```python
from build123d import *

# Parameters (mm, degrees)
BOSS_EXTRUDE1_DEPTH = 177.8
SKETCH4_W           = 153.979316793
SKETCH4_H           = 25.4
BOSS_EXTRUDE4_DEPTH = 177.8
SKETCH3_R           = 73.2155
CUT_EXTRUDE2_DEPTH  = 25.4
FILLET1_R           = 2.54


with BuildPart() as part:
    # Sketch2 → Boss-Extrude1 (new body)
    with BuildSketch(Plane(origin=(0, 0, 0), x_dir=(1, 0, 0), z_dir=(0, 1, 0))):
        Polygon((0, 0), (153.979316793, 0), (153.979316793, 88.9), align=None)
    extrude(amount=BOSS_EXTRUDE1_DEPTH)

    # Sketch4 → Boss-Extrude4 (add)
    with BuildSketch(Plane(origin=(0, 0, 0), x_dir=(-1, 0, 0), z_dir=(0, -1, 0))):
        with Locations((-76.989658397, -12.7)):
            Rectangle(SKETCH4_W, SKETCH4_H)
    extrude(amount=-BOSS_EXTRUDE4_DEPTH)

    # Sketch3 → Cut-Extrude2 (cut)
    with BuildSketch(Plane(origin=(0, 0, 0), x_dir=(-0.8660254037844386, 0, 0.5), z_dir=(-0.5000000000000001, 0, -0.8660254037844387))):
        with Locations((-88.9, 88.9)):
            Circle(SKETCH3_R)
    extrude(amount=-CUT_EXTRUDE2_DEPTH, mode=Mode.SUBTRACT)

    # Fillet1
    fillet1_edges = [part.edges().sort_by_distance(p)[0] for p in [
        (153.979316793, 88.9, 25.4),
        (0, 88.9, 25.4),
        (76.989658396, 0, 25.4),
        (0, 0, 12.7),
        (76.989658396, 177.8, -44.45),
        (0, 177.8, 12.7),
        (76.989658396, 177.8, 25.4),
        (140.396141347, 88.9, -81.05775),
        (76.989658396, 0, -44.45),
        (153.979316793, 0, -31.75),
        (0, 88.9, 0),
        (153.979316793, 88.9, -88.9),
        (153.979316793, 177.8, -31.75),
    ]]
    fillet(fillet1_edges, radius=FILLET1_R)


solid = part.part
```
The model under review builds one solid part; all positions refer to its coordinate system, in mm. Round coordinates to 2 decimals unless told otherwise and drop trailing zeros. Answer as a JSON object with one key per item and string values. Group by question number.
1) Mouldability with a two-part tool opening along Y and no side actions: class faces 1 (the face through (90.577, 89.925, -22.965)), 2 (the face through (97.64, 17.426, -40.426)), 3 (the face through (95, 177.8, -20)), 4 (the face through (95, 0, -20)) as released by +Y, released by -Y, zero draft, split by the parting line, or undercut.
2) For pin 1 Ø1 at (y, z) = (156.5, -65) entering from -X; pin 2 Ø5 at (y, z) = (90.5, -45.5) entering from -X; pin 3 Ø5 at (y, z) = (79, -63) entering from -X, all flat-tipped, find the tip position at first contact; note any pin that passes through.
3) For line 1 (X direction, y = 127, z = -1); line 2 (X direction, y = 116.5, z = 0.5); line 3 (Y direction, x = 56, z = -30), list the stretches that pass through material, from the lowest coordinate up. Write a range as [from, to].
Result set:
{
 "1": {"face 1": "undercut", "face 2": "undercut", "face 3": "released by +Y", "face 4": "released by -Y"},
 "2": {"pin 1": "x = 111.72", "pin 2": "x = 125.28", "pin 3": "x = 148.55"},
 "3": {"line 1": "[1.73, 29.88], [52.53, 153.98]", "line 2": "[0.19, 24.64], [49.93, 153.98]", "line 3": "[0.05, 20.18], [157.62, 177.75]"}
}
